Check sheet for the modelled part. Datum: model origin and axes. Units: mm. Face numbers are marked on the shaded views. A direction names the side the tool comes from. Give positions to 0.01 mm unless a question says otherwise; leave off trailing zeros. Write each loop counter-clockwise with the first axis right and the second up, starting at its lowest first coordinate (ties: lowest second). Pieces come first, ordered by that corner, then holes. Notation, with made-up numbers: M 0,56 L 14,56 A17 ccw 14,84 Z; hole C -14.75,76 d8. An arc over 180 degrees is marked long. Use CSV: the item, a comma, the result in double quotes. Start each with the question number.
1. Access from +Z, -Z, +X, -X, +Y, -Y to the whole of each face (thin tool, end or side, straight path). Record for the marked faces 1, 2 and 3.
2. Cross-section at A-A, the plane z = 1.27. Enter the section's corners in (x, y), and give its area (3 significant figures).
3. Cross-section at C-C, the plane y = 8.75. Enter the section's corners in (x, z).
4. Cross-section at D-D, the plane x = 53.5. Enter the section's corners in (y, z), and give its area (3 significant figures).
5. Scan lines: line 1 (Y direction, x = 1.5, z = 1.27); line 2 (Z direction, x = -45.5, y = 12); line 3 (Y direction, x = -51, z = 0.25). Record each from-to range of solid material in increasing order.
6. Cross-section at B-B, the plane x = -6.5. Enter the section's corners in (y, z), and give its area (3 significant figures).
7. Depth check by flat-ended pin: P1, Ø8, axis at x = -25, y = 7.5, coming from the -Z side; P2, Ø1, axis at x = -3, z = 2, coming from the +Y side; P3, Ø0.8, axis at x = 39, z = 1.5, coming from the +Y side; P4, Ø3, axis at y = 16.9, z = 1.27, coming from the -X side. Enter the tip coordinate at first touch or a pass-through.
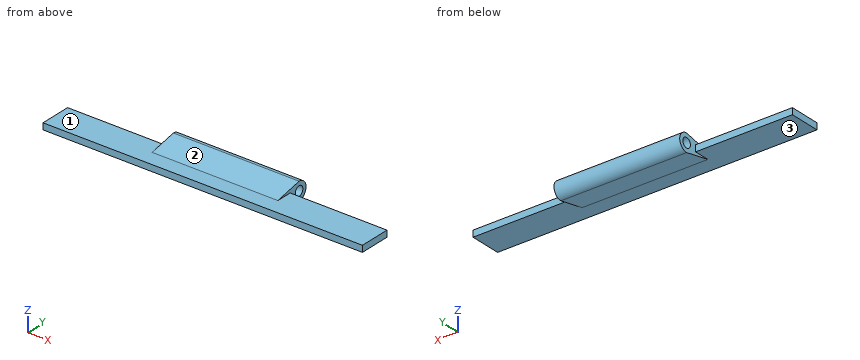
from build123d import *

# Parameters (mm, degrees)
SKETCH1_W           = 127
SKETCH1_H           = 12.4
BOSS_EXTRUDE1_DEPTH = 2.54
SKETCH2_R           = 1.9
BOSS_EXTRUDE3_DEPTH = 25
SKETCH2_2_R         = 1.9
BOSS_EXTRUDE4_DEPTH = 25


with BuildPart() as part:
    # Sketch1 → Boss-Extrude1 (new body)
    with BuildSketch(Plane.XY):
        with Locations((0, 6.2)):
            Rectangle(SKETCH1_W, SKETCH1_H)
    extrude(amount=BOSS_EXTRUDE1_DEPTH)

    # Sketch2 → Boss-Extrude3 (add)
    with BuildSketch(Plane(origin=(0, 0, 0), x_dir=(0, 0, -1), z_dir=(1, 0, 0))):
        with BuildLine():
            Line((-2.54, 6.2), (-4.77, 16.9))
            ThreePointArc((-4.77, 16.9), (-1.27, 20.4), (2.23, 16.9))
            Line((2.23, 16.9), (0, 6.2))
            Line((0, 6.2), (-2.54, 6.2))
        make_face()
        with Locations((-1.27, 16.9)):
            Circle(SKETCH2_R, mode=Mode.SUBTRACT)
    extrude(amount=BOSS_EXTRUDE3_DEPTH)

    # Sketch2_2 → Boss-Extrude4 (add)
    with BuildSketch(Plane(origin=(0, 0, 0), x_dir=(0, 0, -1), z_dir=(1, 0, 0))):
        with BuildLine():
            Line((-2.54, 6.2), (-4.77, 16.9))
            ThreePointArc((-4.77, 16.9), (-1.27, 20.4), (2.23, 16.9))
            Line((2.23, 16.9), (0, 6.2))
            Line((0, 6.2), (-2.54, 6.2))
        make_face()
        with Locations((-1.27, 16.9)):
            Circle(SKETCH2_2_R, mode=Mode.SUBTRACT)
    extrude(amount=-BOSS_EXTRUDE4_DEPTH)


solid = part.part
Worked answers:
1,face 1,"+Z, -Y"
1,face 2,"+Z, +X, -X, -Y"
1,face 3,"-Z, -Y"
2,outline,"M -63.5,0 L 63.5,0 L 63.5,12.4 L 25,12.4 L 25,15 L -25,15 L -25,12.4 L -63.5,12.4 Z; M -25,18.8 L 25,18.8 L 25,20.4 L -25,20.4 Z"
2,area,"1,780 mm^2"
3,outline,"M -63.5,0 L -25,0 L -25,-0.53 L 25,-0.53 L 25,0 L 63.5,0 L 63.5,2.54 L 25,2.54 L 25,3.07 L -25,3.07 L -25,2.54 L -63.5,2.54 Z"
4,outline,"M 0,0 L 12.4,0 L 12.4,2.54 L 0,2.54 Z"
4,area,"31.5 mm^2"
5,line 1,"y = 0 to 15, 18.8 to 20.4"
5,line 2,"z = 0 to 2.54"
5,line 3,"y = 0 to 12.4"
6,outline,"M 0,0 L 6.2,0 L 16.9,-2.23 A3.5 ccw 16.9,4.77 L 6.2,2.54 L 0,2.54 Z; hole C 16.9,1.27 d3.8"
6,area,"74.7 mm^2"
7,P1,"stops at z = -1.1"
7,P2,"stops at y = 20.39"
7,P3,"stops at y = 12.4"
7,P4,"passes through"
